Autodesk Inventor part; units mm, degrees
ref_plane "YZ Plane" through (0, 0, 0) normal (1, 0, 0) x (0, 1, 0)
ref_plane "XZ Plane" through (0, 0, 0) normal (0, 1, 0) x (-1, 0, 0)
ref_plane "XY Plane" through (0, 0, 0) normal (0, 0, 1) x (1, 0, 0)
sketch "Sketch1" plane through (0, 0, 0) normal (0, 1, 0) x (-1, 0, 0)
  line L0 (50.8, 26.924) -> (50.8, -26.924)
  line L1 (6.35, 26.924) -> (6.35, 15.724)
  line L2 (4.85, 14.224) -> (0, 14.224)
  line L3 (6.35, 26.924) -> (50.8, 26.924)
  line L4 (0, -14.224) -> (4.85, -14.224)
  line L5 (6.35, -15.724) -> (6.35, -26.924)
  line L6 (0, 0) -> (0, 14.224)
  line L7 (0, 0) -> (0, -14.224)
  line L8 (6.35, -26.924) -> (50.8, -26.924)
  line L9 (4.85, 14.224) -> (6.35, 15.724)
  line L10 (4.85, -14.224) -> (6.35, -15.724)
  line L11 (50.8, 26.924) -> (50.8, 23.749)
  circle A0 centre (47.625, 23.749) radius 1.524
  line L12 (50.8, -26.924) -> (50.8, -23.749)
  circle A1 centre (47.625, -23.749) radius 1.524
  line L13 (6.35, 26.924) -> (14.478, 26.924)
  circle A2 centre (14.478, 23.749) radius 1.524
  circle A3 centre (3.175, -10.414) radius 1.524
  circle A4 centre (3.175, 10.414) radius 1.524
  point P0 (6.35, 14.224)
  point P1 (6.35, -14.224)
extrude "Extrusion1" add sketch "Sketch1" along normal blind 1
properties part number "Pixy"
Build history of the part. All positions in model axes, mm. Coordinates: 2 decimals unless noted, no trailing zeros. Order: outer loops, then holes, each group sorted by start corner. A loop starts at its lowest first (then second) coordinate and runs counter-clockwise, first axis right, second up. Notation, with made-up numbers: (86, 56) -> (127, 56) arc R12 ccw to (127, 71) -> close; hole circle Ø5 at (79.5, 14). An arc over 180 degrees is marked (long way). One line per item, written item: value.
(1) Slice it at C-C, the plane z = -20. List the corners of the cut face in (x, y).
Checked values:
outline: (-50.8, 0) -> (-6.35, 0) -> (-6.35, 1) -> (-50.8, 1) -> close
(2) Mould opens along Z. For faces 1 (the flat face through (-5.59, 0.493, 14.964)), 2 (the flat face through (-25, 0, 0)), 3 (the cylindrical face through (-46.5, 0.49, 22.72)) say: pulls with the +Z half, pulls with the -Z half, needs draft (parallel to the pull), parting line crosses it, or undercut.
Checked values:
face 1: pulls with the +Z half
face 2: needs draft
face 3: undercut
(3) Probe line 1 (X direction, y = 0.1, z = 24); line 2 (Z direction, x = -49, y = 0.8); line 3 (X direction, y = 0.2, z = 23). List the from-to ranges inside material, lowest first. Write a range as [from, to].
Checked values:
line 1: [-50.8, -49.13], [-46.12, -15.98], [-12.97, -6.35]
line 2: [-26.92, -24.41], [-23.09, 23.09], [24.41, 26.92]
line 3: [-50.8, -48.95], [-46.3, -15.81], [-13.15, -6.35]
(4) Slice it at A-A, the plane x = -14. List the corners of the cut face in (y, z).
Checked values:
outline: (0, -26.92) -> (1, -26.92) -> (1, 22.3) -> (0, 22.3) -> close; (0, 25.2) -> (1, 25.2) -> (1, 26.92) -> (0, 26.92) -> close
(5) Slice it at B-B, the plane y = 0.55. List the corners of the cut face in (x, z) (3 decimals), plus the area to 3 significant figures.
Checked values:
outline: (-50.8, -26.924) -> (-6.35, -26.924) -> (-6.35, -15.724) -> (-4.85, -14.224) -> (0, -14.224) -> (0, 14.224) -> (-4.85, 14.224) -> (-6.35, 15.724) -> (-6.35, 26.924) -> (-50.8, 26.924) -> close; hole circle Ø3.048 at (-47.625, -23.749); hole circle Ø3.048 at (-47.625, 23.749); hole circle Ø3.048 at (-14.478, 23.749); hole circle Ø3.048 at (-3.175, -10.414); hole circle Ø3.048 at (-3.175, 10.414)
area: 2,540 mm2
(6) Drop flat-ended pins along their axis: pin 1 Ø0.5 at (y, z) = (0.5, 21) entering from +X; pin 2 Ø0.5 at (x, y) = (-2.5, 0.5) entering from -Z. Give the stop position or say it passes through.
Checked values:
pin 1: x = -6.35
pin 2: z = -14.22
